CAD build for the part. Positions are in the model's coordinates, mm. Round coordinates to 2 decimals unless told otherwise and drop trailing zeros. Write each loop counter-clockwise with the first axis right and the second up, starting at its lowest first coordinate (ties: lowest second). Pieces come first, ordered by that corner, then holes. Notation, with made-up numbers: (50.25, 18) -> (97.25, 18) arc R16 cw to (97.25, 46) -> close; hole circle Ø8 at (62.25, 23.5). An arc over 180 degrees is marked (long way). Put each result on its own line as item: value. Start each with the question number.
1. Saw through at D-D on x = 4.5. List the corners of the cut face in (y, z).
2. Saw through at C-C on y = 0.4. List the corners of the cut face in (x, z).
3. Flat gauge pin, fed straight in: P1, Ø0.5, axis at x = 28, y = 0.5, coming from the -Z side. Where does the tip first touch, or does it go through?
4. Saw through at B-B on z = -7. List the corners of the cut face in (x, y).
5. Drill centre lines: line 1 (X direction, y = 0.35, z = -7); line 2 (X direction, y = 0.65, z = -8); line 3 (Z direction, x = 22.75, y = 0.9). Where is each one in solid material? Low to high. Write a range as from..to.
6. Saw through at A-A on x = 22.5. List the corners of the cut face in (y, z).
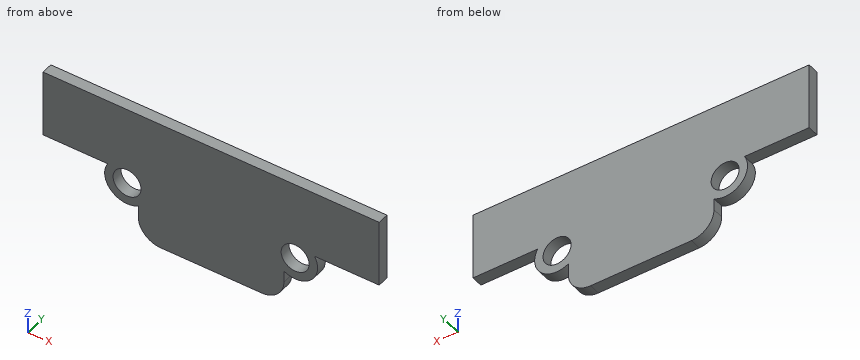
from build123d import *

# Parameters (mm, degrees)
BOSS_EXTRU_1_DEPTH      = 1
ESQUISSE2_R             = 2
BOSS_EXTRU_2_DEPTH      = 1
ESQUISSE3_R             = 1.25
ENL_V_MAT_EXTRU_1_DEPTH = 33.243620766
CONG_1_R                = 2


with BuildPart() as part:
    # Esquisse1 → Boss.-Extru.1 (new body)
    with BuildSketch(Plane(origin=(0, 0, 0), x_dir=(1, 0, 0), z_dir=(0, 1, 0))):
        Polygon((21.5, 6), (30, 6), (30, 0), (0, 0), (0, 6), (8.5, 6), (8.5, 11.775019325), (21.5, 11.775019325), align=None)
    extrude(amount=BOSS_EXTRU_1_DEPTH)

    # Esquisse2 → Boss.-Extru.2 (add)
    with BuildSketch(Plane(origin=(0, 1, 0), x_dir=(1, 0, 0), z_dir=(0, 1, 0))):
        with Locations((7.5, 7)):
            Circle(ESQUISSE2_R)
        with Locations((22.5, 7)):
            Circle(ESQUISSE2_R)
    extrude(amount=-BOSS_EXTRU_2_DEPTH)

    # Esquisse3 → Enlèv. mat.-Extru.1 (cut, through all)
    with BuildSketch(Plane(origin=(0, 1, 0), x_dir=(1, 0, 0), z_dir=(0, 1, 0))):
        with Locations(Location((7.5, 7, 0), (0, 0, 270))):
            Circle(ESQUISSE3_R)
        with Locations(Location((22.5, 7, 0), (0, 0, 270))):
            Circle(ESQUISSE3_R)
    extrude(amount=-ENL_V_MAT_EXTRU_1_DEPTH, mode=Mode.SUBTRACT)

    # Congé1
    cong_1_edges = [part.edges().sort_by_distance(p)[0] for p in [
        (8.5, 0.5, -11.775019325),
        (21.5, 0.5, -11.775019325),
    ]]
    fillet(cong_1_edges, radius=CONG_1_R)


solid = part.part
Return value:
1. outline: (0, -6) -> (1, -6) -> (1, 0) -> (0, 0) -> close
2. outline: (0, -6) -> (5.77, -6) arc R2 ccw to (8.5, -8.73) -> (8.5, -9.78) arc R2 ccw to (10.5, -11.78) -> (19.5, -11.78) arc R2 ccw to (21.5, -9.78) -> (21.5, -8.73) arc R2 ccw to (24.23, -6) -> (30, -6) -> (30, 0) -> (0, 0) -> close; hole circle Ø2.5 at (7.5, -7); hole circle Ø2.5 at (22.5, -7)
3. P1: stops at z = -6
4. outline: (5.5, 0) -> (6.25, 0) -> (6.25, 1) -> (5.5, 1) -> close; (8.75, 0) -> (21.25, 0) -> (21.25, 1) -> (8.75, 1) -> close; (23.75, 0) -> (24.5, 0) -> (24.5, 1) -> (23.75, 1) -> close
5. line 1: x = 5.5..6.25, 8.75..21.25, 23.75..24.5
5. line 2: x = 5.77..6.75, 8.25..21.75, 23.25..24.23
5. line 3: z = -8.98..-8.22, -5.78..0
6. outline: (0, -9) -> (1, -9) -> (1, -8.25) -> (0, -8.25) -> close; (0, -5.75) -> (1, -5.75) -> (1, 0) -> (0, 0) -> close
